Could you check a few things on this drawing? It's one solid part, dimensions in mm from its lowest x, y, z. A direction names the side the tool comes from. Give positions to 0.01 mm unless a question says otherwise; leave off trailing zeros. Loops run counter-clockwise (first coordinate to the right, second up) from the corner with the lowest first, then second, coordinate; pieces in that order, holes last. Notation, with made-up numbers: M 58,72 L 93,72 A28 ccw 93,98 Z; hole C 84.25,62 d1. An arc over 180 degrees is marked long. Return JSON: item names as keys, results as strings. Group by question number.
1. If we section it at C-C (z = 40): Write out the boundary of the cut face in (x, y).
2. If we mould it in two halves opening along Y, with no side actions, what happens to the marked faces 3, 4 and 5? For each: +Y half, -Y half, draft (parallel to the pull), parting line (faces both ways), or undercut.
3. If we section it at A-A (y = 85): Write out the boundary of the cut face in (x, z).
4. If we section it at D-D (y = 67.5): Write out the boundary of the cut face in (x, z), plus the area to 3 significant figures.
5. For pin 1 (11 mm diameter, centred on y = 15, z = 40, fed in from +X); pin 2 (11 mm diameter, centred on y = 12.5, z = 42, fed in from +X); pin 3 (3 mm diameter, centred on x = 54.5, z = 46, fed in from +Y), each with a flat end and sliding along its axis, tell me the tip position at first contact or that it passes through.
6. Please list where these lines run through material, in increasing order: line 1 (Y direction, x = 55.5, z = 40); line 2 (Z direction, x = 58, y = 85); line 3 (X direction, y = 30, z = 42).
7. If we section it at B-B (x = 63.5): Write out the boundary of the cut face in (y, z), plus the area to 3 significant figures.
8. For the marked faces 1 and 2, which set-ups out of +Z, -Z, +X, -X, +Y, -Y let a thin tool reach every point of the face, with its end or its side?
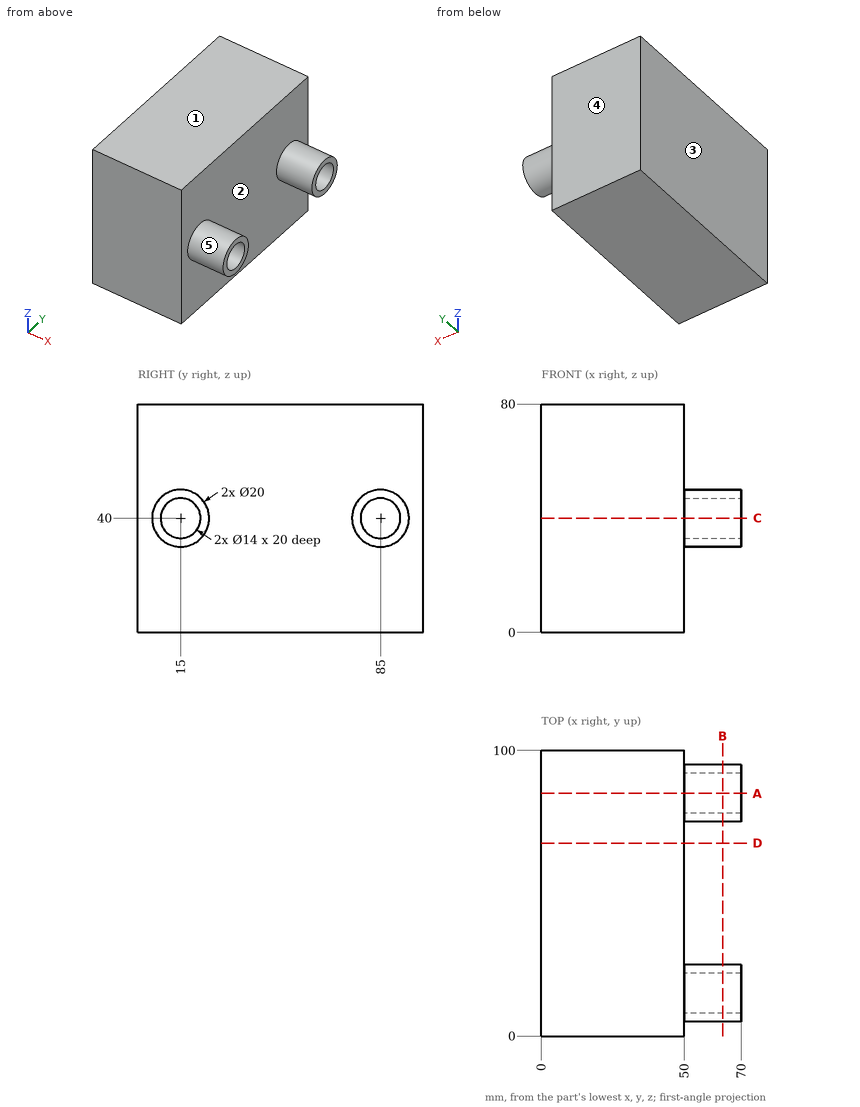
Answer:
{
 "1": {"outline": "M 0,0 L 50,0 L 50,5 L 70,5 L 70,8 L 50,8 L 50,22 L 70,22 L 70,25 L 50,25 L 50,75 L 70,75 L 70,78 L 50,78 L 50,92 L 70,92 L 70,95 L 50,95 L 50,100 L 0,100 Z"},
 "2": {"face 3": "draft", "face 4": "+Y half", "face 5": "undercut"},
 "3": {"outline": "M 0,0 L 50,0 L 50,30 L 70,30 L 70,33 L 50,33 L 50,47 L 70,47 L 70,50 L 50,50 L 50,80 L 0,80 Z"},
 "4": {"outline": "M 0,0 L 50,0 L 50,80 L 0,80 Z", "area": "4,000 mm²"},
 "5": {"pin 1": "stops at x = 50", "pin 2": "stops at x = 70", "pin 3": "stops at y = 93.93"},
 "6": {"line 1": "y = 5 to 8, 22 to 25, 75 to 78, 92 to 95", "line 2": "z = 30 to 33, 47 to 50", "line 3": "x = 0 to 50"},
 "7": {"outline": "C 15,40 d20; C 85,40 d20; hole C 15,40 d14; hole C 85,40 d14", "area": "320 mm²"},
 "8": {"face 1": "+Z, +X, -X, +Y, -Y", "face 2": "+X"}
}
